Input: part model. Units: mm. Frame: model coordinates. A direction names the side the tool comes from. Give positions to 0.01 mm unless a question says otherwise; leave off trailing zeros. Loops run counter-clockwise (first coordinate to the right, second up) from the corner with the lowest first, then second, coordinate; pieces in that order, holes last. Notation, with made-up numbers: (9.25, 3.25) -> (42.25, 3.25) arc R24 cw to (42.25, 32.25) -> close; hole circle Ø8 at (66, 89.25). An arc over 180 degrees is marked (long way). Answer as a JSON object with one key per item and string values. Group by question number.
```python
from build123d import *

# Parameters (mm, degrees)
BOSS_EXTRUDE1_DEPTH  = 15
M3_CLEARANCE_HOLE1_D = 3.2
BOSS_EXTRUDE2_DEPTH  = 3.5
M2_CLEARANCE_HOLE2_D = 2.2
SKETCH8_R            = 1.45
BOSS_EXTRUDE3_DEPTH  = 4
SKETCH8_3_R          = 1.45
CUT_EXTRUDE1_DEPTH   = 3
FILLET3_R            = 0.5
SKETCH11_R           = 8.1
CUT_EXTRUDE3_DEPTH   = 15


with BuildPart() as part:
    # Sketch1 → Boss-Extrude1 (new body)
    with BuildSketch(Plane.XY):
        with BuildLine():
            Line((-8, 0), (-14, 0))
            Line((-14, 0), (-14, 12))
            Line((-14, 12), (14, 12))
            Line((14, 12), (14, 0))
            Line((14, 0), (8, 0))
            ThreePointArc((8, 0), (0, 8), (-8, 0))
        make_face()
    extrude(amount=-BOSS_EXTRUDE1_DEPTH)

    # M3 Clearance Hole1 (through all)
    with Locations(Plane(origin=(0, 0, 0), x_dir=(-1, 0, 0), z_dir=(0, -1, 0))):
        with Locations((11, 11), (11, 4), (-11, 11), (-11, 4)):
            Hole(M3_CLEARANCE_HOLE1_D / 2)

    # Sketch5 → Boss-Extrude2 (add)
    with BuildSketch(Plane.XY):
        with BuildLine():
            Line((-3.5, 0), (-14, 0))
            Line((-14, 0), (-14, 12))
            Line((-14, 12), (14, 12))
            Line((14, 12), (14, 0))
            Line((14, 0), (3.5, 0))
            ThreePointArc((3.5, 0), (0, 3.5), (-3.5, 0))
        make_face()
    extrude(amount=BOSS_EXTRUDE2_DEPTH)

    # M2 Clearance Hole2 (through all)
    with Locations(Plane.XY.offset(3.5)):
        with Locations((0, 5.25)):
            Hole(M2_CLEARANCE_HOLE2_D / 2)

    # Sketch8 → Boss-Extrude3 (add)
    with BuildSketch(Plane.XY.offset(3.5)):
        with BuildLine():
            Line((-14, 12.5), (-14, 12))
            Line((-14, 12), (-0.734846923, 12))
            ThreePointArc((-0.734846923, 12), (-0.720059707, 14.508576187), (1.45, 13.25))
            ThreePointArc((1.45, 13.25), (1.258576187, 12.529940293), (0.734846923, 12))
            Line((0.734846923, 12), (14, 12))
            Line((14, 12), (14, 12.5))
            ThreePointArc((14, 12.5), (7.683135649, 13.42711883), (1.899082569, 16.130275229))
            ThreePointArc((1.899082569, 16.130275229), (0, 16.7), (-1.899082569, 16.130275229))
            ThreePointArc((-1.899082569, 16.130275229), (-7.683135649, 13.42711883), (-14, 12.5))
        make_face()
        with Locations((0, 13.25)):
            Circle(SKETCH8_R)
    extrude(amount=-BOSS_EXTRUDE3_DEPTH)

    # Sketch8<3> → Cut-Extrude1 (cut)
    with BuildSketch(Plane.XY.offset(3.5)):
        with Locations((0, 13.25)):
            Circle(SKETCH8_3_R)
        with BuildLine():
            ThreePointArc((1.45, 13.25), (-0.720059707, 14.508576187), (-0.734846923, 12))
            Line((-0.734846923, 12), (0.734846923, 12))
            ThreePointArc((0.734846923, 12), (1.258576187, 12.529940293), (1.45, 13.25))
        make_face()
        with BuildLine():
            Line((0.734846923, 12), (-0.734846923, 12))
            ThreePointArc((-0.734846923, 12), (0, 11.8), (0.734846923, 12))
        make_face()
    extrude(amount=-CUT_EXTRUDE1_DEPTH, mode=Mode.SUBTRACT)

    # Fillet3
    fillet3_edges = [part.edges().sort_by_distance(p)[0] for p in [
        (-14, 12, -7.75),
        (14, 12, -7.75),
        (14, 6, -15),
        (0, 12, -15),
        (-14, 6, -15),
        (14, 6.25, 3.5),
        (-14, 6.25, 3.5),
        (14, 12.5, 1.5),
        (-14, 12.5, 1.5),
    ]]
    fillet(fillet3_edges, radius=FILLET3_R)

    # Sketch11 → Cut-Extrude3 (cut)
    with BuildSketch(Plane(origin=(0, 0, -15), x_dir=(-1, 0, 0), z_dir=(0, 0, -1))):
        Circle(SKETCH11_R)
    extrude(amount=-CUT_EXTRUDE3_DEPTH, mode=Mode.SUBTRACT)


solid = part.part
```
Q1. Pin query (flat end, axial travel): pin 1 Ø0.9 at (x, y) = (0.5, 13.5) entering from +Z; pin 2 Ø2.5 at (x, z) = (11, -4) entering from -Y; pin 3 Ø1.6 at (x, y) = (-6, 13) entering from -Z; pin 4 Ø7 at (x, z) = (5.5, -6.5) entering from +Y. Return the tip coordinate at first contact, or that it passes through.
Q2. Section C-C on z = -8.25. Return the cut outline in (x, y), then the cut area to 3 significant figures.
Q3. Section A-A on x = 0. Return the cut outline in (y, z), then the cut area to 3 significant figures.
Q4. Section D-D on y = 7.25. Return the cut outline in (x, z), then the cut area to 3 significant figures.
Q5. Section B-B on y = 5.25. Return the cut outline in (x, z), then the cut area to 3 significant figures.
Q6. Pull-direction query (Y, two-part tool) for faces 1 (the face through (-0.59, 6.18, 1.73)), 2 (the face through (0, 13, 0.5)), 3 (the face through (0, 16.7, 1.5)), 4 (the face through (-12.6, 6.08, -11.07)); classes: +Y half, -Y half, draft (parallel to the pull), parting line (faces both ways), or undercut.
Q7. Ray query, probe 1 along Z at (x, y) = (11, 8.25); probe 2 along X at (y, z) = (9.5, -11); probe 3 along Y at (x, z) = (0, 1.5). Return the intervals inside material, ascending.
Q8. Set-up query: faces 5 (the face through (0.2, 8.4, -15)), 6 (the face through (0, 12, -8)). Return all of +Z, -Z, +X, -X, +Y, -Y with unobstructed straight access to the full face (end or side cutting, diameter ignored); none if empty.
Numbers:
{
 "1": {"pin 1": "stops at z = 0.5", "pin 2": "passes through", "pin 3": "stops at z = -0.5", "pin 4": "stops at y = 12"},
 "2": {"outline": "(-14, 0) -> (-8.1, 0) arc R8.1 cw to (8.1, 0) -> (14, 0) -> (14, 11.5) arc R0.5 ccw to (13.5, 12) -> (-13.5, 12) arc R0.5 ccw to (-14, 11.5) -> close", "area": "233 mm²"},
 "3": {"outline": "(3.5, 0) -> (4.15, 0) -> (4.15, 3.5) -> (3.5, 3.5) -> close; (6.35, 0) -> (8.1, 0) -> (8.1, -15) -> (11.5, -15) arc R0.5 ccw to (12, -14.5) -> (12, -0.5) -> (16.7, -0.5) -> (16.7, 3.5) -> (14.7, 3.5) -> (14.7, 0.5) -> (11.8, 0.5) -> (11.8, 3.5) -> (6.35, 3.5) -> close", "area": "90.6 mm²"},
 "4": {"outline": "(-14, -14.5) arc R0.5 ccw to (-13.5, -15) -> (-3.61, -15) -> (-3.61, 0) -> (3.61, 0) -> (3.61, -15) -> (13.5, -15) arc R0.5 ccw to (14, -14.5) -> (14, 3) arc R0.5 ccw to (13.5, 3.5) -> (-13.5, 3.5) arc R0.5 ccw to (-14, 3) -> close; hole circle Ø3.2 at (-11, -11); hole circle Ø3.2 at (-11, -4); hole circle Ø3.2 at (11, -11); hole circle Ø3.2 at (11, -4)", "area": "377 mm²"},
 "5": {"outline": "(-14, -14.5) arc R0.5 ccw to (-13.5, -15) -> (-6.17, -15) -> (-6.17, 0) -> (-1.1, 0) -> (-1.1, 3.5) -> (-13.5, 3.5) arc R0.5 ccw to (-14, 3) -> close; (1.1, 0) -> (6.17, 0) -> (6.17, -15) -> (13.5, -15) arc R0.5 ccw to (14, -14.5) -> (14, 3) arc R0.5 ccw to (13.5, 3.5) -> (1.1, 3.5) -> close; hole circle Ø3.2 at (-11, -11); hole circle Ø3.2 at (-11, -4); hole circle Ø3.2 at (11, -11); hole circle Ø3.2 at (11, -4)", "area": "293 mm²"},
 "6": {"face 1": "undercut", "face 2": "undercut", "face 3": "+Y half", "face 4": "draft"},
 "7": {"probe 1": "z = -15 to -12.6, -9.4 to -5.6, -2.4 to 3.5", "probe 2": "x = -14 to -12.6, -9.4 to 9.4, 12.6 to 14", "probe 3": "y = 3.5 to 4.15, 6.35 to 11.8, 14.7 to 16.7"},
 "8": {"face 5": "-Z, +X, -X, +Y, -Y", "face 6": "-Z, +X, -X, +Y"}
}
